Part model, mm, in its own coordinate system. Coordinates: 2 decimals unless noted, no trailing zeros. Order: outer loops, then holes, each group sorted by start corner. A loop starts at its lowest first (then second) coordinate and runs counter-clockwise, first axis right, second up.
1) Cut at D-D (z = -134.5). List the corners of the cut face in (x, y), and give its area (3 significant figures).
2) Cut at B-B (y = 289.2). List the corners of the cut face in (x, z), and give its area (3 significant figures).
3) Cut at A-A (z = -67.5). List the corners of the cut face in (x, y), and give its area (3 significant figures).
4) Cut at C-C (x = 7). Give the number of separate pieces and of enclosed holes in the cut face, and give its area (3 significant figures).
5) Pin check, flat tips, straight feed: pin 1 Ø3 at (x, z) = (4.5, -86) entering from +Y; pin 2 Ø6 at (x, y) = (3.5, 233.5) entering from -Z; pin 3 Ø6 at (x, y) = (7.5, 342) entering from -Z. Stop position of each tip, or through.
6) Wall check: L1, parallel to Y at x = 1, z = -75; L2, parallel to Y at x = 1.25, z = -61; L3, parallel to Z at x = 8.75, y = 222. Give the ranges that are in metal, low to high.
```python
from build123d import *

# Parameters (mm, degrees)
CROQUIS1_R              = 3
CROQUIS1_R_2            = 20
CROQUIS1_R_3            = 3.425181835
CROQUIS1_W              = 12.7
CROQUIS1_H              = 50.8
SALIENTE_EXTRUIR1_DEPTH = 12


with BuildPart() as part:
    # Croquis1 → Saliente-Extruir1 (new body)
    with BuildSketch(Plane(origin=(0, 0, 0), x_dir=(0, 0, -1), z_dir=(1, 0, 0))):
        with BuildLine():
            Line((0, 0), (0, 380))
            ThreePointArc((0, 380), (5.857864376, 394.142135624), (20, 400))
            Line((20, 400), (82.802037251, 400))
            ThreePointArc((82.802037251, 400), (95.841934647, 395.164467544), (102.576347335, 382.996107589))
            Line((102.576347335, 382.996107589), (149.774310084, 71.489553442))
            ThreePointArc((149.774310084, 71.489553442), (149.943497708, 69.995743812), (150, 68.493445854))
            Line((150, 68.493445854), (150, 0))
            Line((150, 0), (0, 0))
        make_face()
        with Locations((30, 45)):
            Circle(CROQUIS1_R, mode=Mode.SUBTRACT)
        with Locations((60, 45)):
            Circle(CROQUIS1_R, mode=Mode.SUBTRACT)
        with Locations((90, 45)):
            Circle(CROQUIS1_R, mode=Mode.SUBTRACT)
        with Locations((120, 45)):
            Circle(CROQUIS1_R, mode=Mode.SUBTRACT)
        with Locations((30, 15)):
            Circle(CROQUIS1_R, mode=Mode.SUBTRACT)
        with Locations((60, 15)):
            Circle(CROQUIS1_R, mode=Mode.SUBTRACT)
        with Locations((90, 15)):
            Circle(CROQUIS1_R, mode=Mode.SUBTRACT)
        with Locations((120, 15)):
            Circle(CROQUIS1_R, mode=Mode.SUBTRACT)
        with Locations((32.7, 289.2)):
            Circle(CROQUIS1_R_2, mode=Mode.SUBTRACT)
        with Locations((12.273774242, 309.320061608)):
            Circle(CROQUIS1_R_3, mode=Mode.SUBTRACT)
        with Locations((53.126225758, 309.320061608)):
            Circle(CROQUIS1_R_3, mode=Mode.SUBTRACT)
        with Locations((53.126225758, 269.079938392)):
            Circle(CROQUIS1_R_3, mode=Mode.SUBTRACT)
        with Locations((12.273774242, 269.079938392)):
            Circle(CROQUIS1_R_3, mode=Mode.SUBTRACT)
        with Locations((26.35, 354.6)):
            Rectangle(CROQUIS1_W, CROQUIS1_H, mode=Mode.SUBTRACT)
        with Locations((26.35, 223.8)):
            Rectangle(CROQUIS1_W, CROQUIS1_H, mode=Mode.SUBTRACT)
        with BuildLine():
            Line((60, 90), (83.2545966, 90))
            ThreePointArc((83.2545966, 90), (98.419064144, 96.960102603), (103.028906685, 112.996107589))
            Line((103.028906685, 112.996107589), (98.483452139, 142.996107589))
            ThreePointArc((98.483452139, 142.996107589), (91.749039451, 155.164467544), (78.709142055, 160))
            Line((78.709142055, 160), (60, 160))
            ThreePointArc((60, 160), (45.857864376, 154.142135624), (40, 140))
            Line((40, 140), (40, 110))
            ThreePointArc((40, 110), (45.857864376, 95.857864376), (60, 90))
        make_face(mode=Mode.SUBTRACT)
    extrude(amount=SALIENTE_EXTRUIR1_DEPTH)


solid = part.part
```
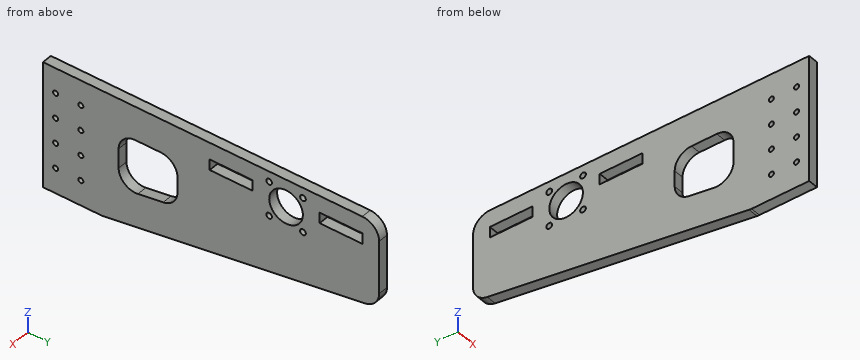
Geometry check:
1. outline: (0, 0) - (12, 0) - (12, 172.3) - (0, 172.3) - close
1. area: 2,070 mm2
2. outline: (0, -116.79) - (12, -116.79) - (12, -52.7) - (0, -52.7) - close; (0, -12.7) - (12, -12.7) - (12, 0) - (0, 0) - close
2. area: 921 mm2
3. outline: (0, 0) - (12, 0) - (12, 90) - (0, 90) - close; (0, 160) - (12, 160) - (12, 400) - (0, 400) - close
3. area: 3,960 mm2
4. separate pieces: 1
4. enclosed holes: 16
4. area: 44,800 mm2
5. pin 1: stops at y = 399.93
5. pin 2: stops at z = -125.68
5. pin 3: stops at z = -109.24
6. L1: y = 0 to 90, 160 to 400
6. L2: y = 0 to 12.17, 17.83 to 42.17, 47.83 to 90, 160 to 400
6. L3: z = -126.97 to -32.7, -20 to 0
